Part model, mm, in its own coordinate system. A direction names the side the tool comes from. Round coordinates to 2 decimals unless told otherwise and drop trailing zeros. Write each loop counter-clockwise with the first axis right and the second up, starting at its lowest first coordinate (ties: lowest second). Pieces come first, ordered by that corner, then holes.
from build123d import *

# Parameters (mm, degrees)
F0_W      = 70
F0_H      = 54
F1_DEPTH  = 23
F3_DEPTH  = 60
F4_W      = 64
F4_H      = 48
F5_DEPTH  = 15
F6_R      = 2
F7_DEPTH  = 25
F9_DEPTH  = 25
F11_DEPTH = 25
F12_W     = 1.5
F12_H     = 36
F12_W_2   = 13.280427
F12_H_2   = 3
F12_W_3   = 51
F12_W_4   = 12.749882
F12_W_5   = 3
F12_H_3   = 49.144776
F12_H_4   = 1.5
F12_H_5   = 10.144776
F12_W_6   = 67.280427
F12_W_7   = 66.749882
F13_DEPTH = 8


with BuildPart() as f1:
    # F0 (on Top) → F1 (new body)
    with BuildSketch(Plane.XY):
        Rectangle(F0_W, F0_H)
    extrude(amount=-F1_DEPTH)

    # F2 (on face) → F3 (cut)
    with BuildSketch(Plane.XZ.offset(27)):
        with BuildLine():
            Line((-35, -23), (35, -23))
            ThreePointArc((35, -23), (0, -18), (-35, -23))
        make_face()
    extrude(amount=-F3_DEPTH, mode=Mode.SUBTRACT)

    # F4 (on face) → F5 (cut)
    with BuildSketch(Plane.XY):
        Rectangle(F4_W, F4_H)
    extrude(amount=-F5_DEPTH, mode=Mode.SUBTRACT)

    # F6 (on face) → F7 (cut)
    with BuildSketch(Plane.XY.offset(-15)):
        with Locations((-27, 19.5)):
            Circle(F6_R)
        with Locations((-27, -19.5)):
            Circle(F6_R)
        with Locations((27, -19.5)):
            Circle(F6_R)
        with Locations((27, 19.5)):
            Circle(F6_R)
    extrude(amount=-F7_DEPTH, mode=Mode.SUBTRACT)

    # F8 (on face) → F9 (cut)
    with BuildSketch(Plane.XY.offset(-15)):
        Polygon((37, 6), (32, 6), (32, -15), (38.883269, -15), (38.883269, 6), align=None)
    extrude(amount=F9_DEPTH, mode=Mode.SUBTRACT)

    # F10 (on face) → F11 (cut)
    with BuildSketch(Plane.XY.offset(-15)):
        Polygon((8, -24), (-10, -24), (-10, -27.841958), (-10, -32.821599), (8, -32.821599), align=None)
    extrude(amount=F11_DEPTH, mode=Mode.SUBTRACT)

    # F12 (on face) → F13 (cut)
    with BuildSketch(Plane.XY.offset(-15)):
        with Locations((27.75, 0)):
            Rectangle(F12_W, F12_H)
        Polygon((25.5, 18), (27, 18), (28.5, 18), (28.5, 21), (25.5, 21), align=None)
        with Locations((35.140214, 19.5)):
            Rectangle(F12_W_2, F12_H_2)
        with Locations((0, 19.5)):
            Rectangle(F12_W_3, F12_H_2)
        with Locations((34.874941, -19.5)):
            Rectangle(F12_W_4, F12_H_2)
        with Locations((27, 45.572388)):
            Rectangle(F12_W_5, F12_H_3)
        Polygon((-27, 18), (-25.5, 18), (-25.5, 21), (-28.5, 21), (-28.5, 18), align=None)
        with Locations((0, -20.25)):
            Rectangle(F12_W_3, F12_H_4)
        with Locations((27, -26.072388)):
            Rectangle(F12_W_5, F12_H_5)
        with Locations((-27, 45.572388)):
            Rectangle(F12_W_5, F12_H_3)
        with Locations((-27.75, 0)):
            Rectangle(F12_W, F12_H)
        with Locations((-62.140213, 19.5)):
            Rectangle(F12_W_6, F12_H_2)
        with Locations((-27, -26.072388)):
            Rectangle(F12_W_5, F12_H_5)
        with Locations((-61.874941, -19.5)):
            Rectangle(F12_W_7, F12_H_2)
    extrude(amount=F13_DEPTH, mode=Mode.SUBTRACT)


solid = f1.part
Q1. Tool access for faces 3 (the flat face through (-28.5, -26, -11)), 4 (the flat face through (-21, -24, -7)), 5 (the flat face through (33, 21, -11)): list every direction of +Z, -Z, +X, -X, +Y, -Y with a clear straight run to the whole face (end or side of a thin tool).
Q2. Drop flat-ended pins along their axis: P1, Ø1.5, axis at x = 26.5, y = 26, coming from the -Z side; P2, Ø2, axis at x = -14, y = -6, coming from the -Z side; P3, Ø5, axis at y = 2.5, z = -5.5, coming from the +X side. Give the stop position or say it passes through.
Q3. Saw through at D-D, the plane y = -6. Write the cut outline in (x, z), and give its area (3 significant figures).
Q4. Wall check: line 1 (Y direction, x = 27, z = -19); line 2 (X direction, y = 17, z = -4.5); line 3 (Y direction, x = 7.5, z = -1). Give the ranges that are in metal, low to high.
Q5. Saw through at A-A, the plane z = -2. Write the cut outline in (x, y), and give its area (3 significant figures).
Q6. Two-plate mould, pull along Z, no slides. Class faces 1 (the flat face through (32, 15, -7)), 2 (the flat face through (-34, -18, -11)): released by +Z, released by -Z, zero draft, split by the parting line, or undercut.
Q7. Saw through at C-C, the plane x = -27. Write the cut outline in (y, z).
Q8. Saw through at B-B, the plane y = -19.5. Write the cut outline in (x, z), and give its area (3 significant figures).
Computed:
1. face 3: +Y, -Y
1. face 4: +Z
1. face 5: +X, -X
2. P1: stops at z = -21.01
2. P2: stops at z = -18.9
2. P3: stops at x = -32
3. outline: (-35, -23) arc R125 cw to (35, -23) - (35, -15) - (-32, -15) - (-32, 0) - (-35, 0) - close
3. area: 371 mm2
4. line 1: y = -27 to -21.5, -17.5 to 17.5, 21.5 to 27
4. line 2: x = -35 to -32, 32 to 35
4. line 3: y = 24 to 27
5. outline: (-35, -27) - (-10, -27) - (-10, -24) - (-32, -24) - (-32, 24) - (32, 24) - (32, 6) - (35, 6) - (35, 27) - (-35, 27) - close; (8, -27) - (35, -27) - (35, -15) - (32, -15) - (32, -24) - (8, -24) - close
5. area: 591 mm2
6. face 1: zero draft
6. face 2: undercut
7. outline: (-27, -20.95) - (-21.5, -20.95) - (-21.5, -15) - (-27, -15) - close; (-27, -7) - (-24, -7) - (-24, 0) - (-27, 0) - close; (-17.5, -20.95) - (17.5, -20.95) - (17.5, -15) - (-17.5, -15) - close; (21.5, -20.95) - (27, -20.95) - (27, -15) - (21.5, -15) - close; (24, -7) - (27, -7) - (27, 0) - (24, 0) - close
8. outline: (-35, -23) arc R125 cw to (-29, -21.41) - (-29, -15) - (-35, -15) - close; (-35, -7) - (-32, -7) - (-32, 0) - (-35, 0) - close; (-25, -20.53) arc R125 cw to (25, -20.53) - (25, -15) - (-25, -15) - close; (29, -21.41) arc R125 cw to (35, -23) - (35, -15) - (29, -15) - close; (32, -7) - (35, -7) - (35, 0) - (32, 0) - close
8. area: 320 mm2
